Could you check a few things on this drawing? It's one solid part, dimensions in mm from its lowest x, y, z. A direction names the side the tool comes from. Round coordinates to 2 decimals unless told otherwise and drop trailing zeros. Loops run counter-clockwise (first coordinate to the right, second up) from the corner with the lowest first, then second, coordinate; pieces in that order, holes last.
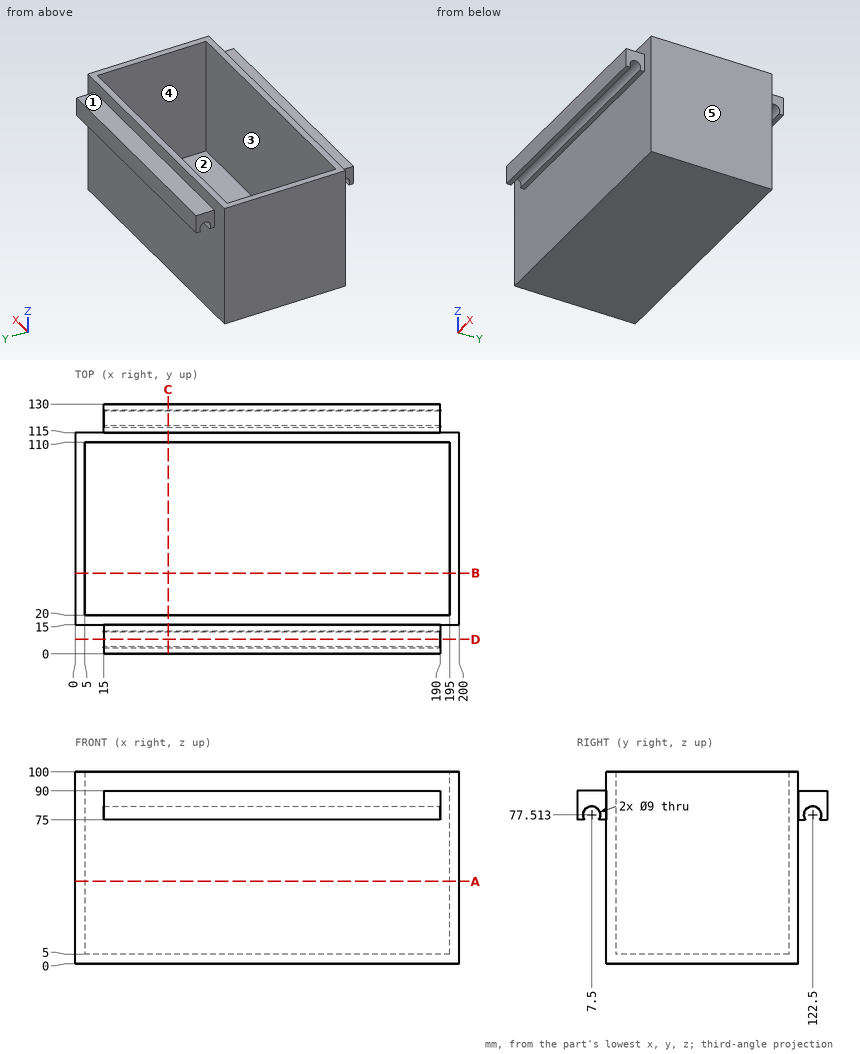
(1) Suppose I cut it at A-A (z = 43). Write out the boundary of the cut face in (x, y), then the cut area to 3 significant figures.
(2) If I drill on line 1 (Y direction, x = 169, z = 73); line 2 (X direction, y = 65, z = 9); line 3 (Y direction, x = 29.5, z = 89), over which ranges is the centre line in solid material (lowest first)?
(3) Which directions (+Z, -Z, +X, -X, +Y, -Y) give clear straight access to the entire face, cutting with the end or side of a thin tool? Please do the marked faces 4 and 5.
(4) We'd pull the mould along Y, two halves only. Please class the marked faces 1, 2 and 3: released by +Y, released by -Y, zero draft, split by the parting line, or undercut.
(5) Suppose I cut it at C-C (x = 48.5). Write out the boundary of the cut face in (y, z).
(6) Suppose I cut it at D-D (y = 7.5). Write out the boundary of the cut face in (x, z).
(7) For pin 1 (4.5 mm diameter, centred on y = 9.5, z = 82, fed in from +X); pin 2 (1 mm diameter, centred on y = 29.5, z = 74.5, fed in from -X); pin 3 (1.1 mm diameter, centred on x = 97.5, y = 13.5, fed in from -Z); pin 4 (8 mm diameter, centred on y = 7.5, z = 77.51, fed in from +X), each with a flat end and sliding along its axis, tell me the tip position at first contact or that it passes through.
(8) Suppose I cut it at B-B (y = 42). Write out the boundary of the cut face in (x, z).
Check result:
1. outline: (0, 15) - (200, 15) - (200, 115) - (0, 115) - close; hole (5, 20) - (195, 20) - (195, 110) - (5, 110) - close
1. area: 2,900 mm2
2. line 1: y = 15 to 20, 110 to 115
2. line 2: x = 0 to 5, 195 to 200
2. line 3: y = 0 to 20, 110 to 130
3. face 4: +Z
3. face 5: +Z, -Z, +X, +Y, -Y
4. face 1: zero draft
4. face 2: undercut
4. face 3: undercut
5. outline: (0, 75) - (3.77, 75) arc R4.5 cw (long way) to (11.23, 75) - (15, 75) - (15, 0) - (115, 0) - (115, 75) - (118.77, 75) arc R4.5 cw (long way) to (126.23, 75) - (130, 75) - (130, 90) - (115, 90) - (115, 100) - (110, 100) - (110, 5) - (20, 5) - (20, 100) - (15, 100) - (15, 90) - (0, 90) - close
6. outline: (15, 82.01) - (190, 82.01) - (190, 90) - (15, 90) - close
7. pin 1: stops at x = 190
7. pin 2: stops at x = 0
7. pin 3: stops at z = 75
7. pin 4: passes through
8. outline: (0, 0) - (200, 0) - (200, 100) - (195, 100) - (195, 5) - (5, 5) - (5, 100) - (0, 100) - close
